Geometry check sheet. Reference: the model listing, model coordinates, mm. Face numbers are marked on the shaded views. A direction names the side the tool comes from. Give positions to 0.01 mm unless a question says otherwise; leave off trailing zeros. Order: outer loops, then holes, each group sorted by start corner. A loop starts at its lowest first (then second) coordinate and runs counter-clockwise, first axis right, second up. Notation, with made-up numbers: (65, 17) - (119, 17) arc R18 ccw to (119, 52) - close; hole circle Ø6 at (44, 24). An arc over 180 degrees is marked (long way). Put each result on its own line as item: value. Start each with the question number.
```python
from build123d import *

# Parameters (mm, degrees)
SKETCH1_W           = 40.5
SKETCH1_H           = 28.26
BOSS_EXTRUDE1_DEPTH = 2
SKETCH2_R           = 44
CUT_EXTRUDE1_DEPTH  = 1.8
CHAMFER1_SIZE       = 4.945459355
CHAMFER1_SIZE_2     = 1.8
CUT_EXTRUDE2_DEPTH  = 43.940737069


with BuildPart() as part:
    # Sketch1 → Boss-Extrude1 (new body)
    with BuildSketch(Plane(origin=(0, 0, 0), x_dir=(1, 0, 0), z_dir=(0, 1, 0))):
        Rectangle(SKETCH1_W, SKETCH1_H)
    extrude(amount=BOSS_EXTRUDE1_DEPTH)

    # Sketch2 → Cut-Extrude1 (cut)
    with BuildSketch(Plane(origin=(0, 2, 0), x_dir=(1, 0, 0), z_dir=(0, 1, 0))):
        with Locations((0, 51.13)):
            Circle(SKETCH2_R)
    extrude(amount=-CUT_EXTRUDE1_DEPTH, mode=Mode.SUBTRACT)

    # Chamfer1
    # the kernel refuses this chamfer: 4.945459355, 1.8 mm, written as the material it takes off along each edge
    with BuildSketch(Plane(origin=(0, 2, -51.13), x_dir=(-0.6960446295726113, 0, 0.7179985192485611), z_dir=(-0.7179985192485611, 0, -0.6960446295726113))) as chamfer1_piece_1_section:
        Polygon((44 + CHAMFER1_SIZE, 0), (44, -CHAMFER1_SIZE_2), (44, 0), align=None)
    chamfer1_piece_1 = revolve(axis=Axis((0, 2, -51.13), (0, 1, 0)), revolution_arc=88.221038487, mode=Mode.PRIVATE)
    chamfer1_piece_1 = split(chamfer1_piece_1, bisect_by=Plane(origin=(0, 0.2, -4.588848893), z_dir=(0, 1, 0)), keep=Keep.TOP, mode=Mode.PRIVATE)
    add(chamfer1_piece_1, mode=Mode.SUBTRACT)

    # Sketch3 → Cut-Extrude2 (cut, through all)
    with BuildSketch(Plane(origin=(20.25, 0, 0), x_dir=(0, 0, -1), z_dir=(1, 0, 0))):
        Polygon((-12.38, 2), (-11.63, 1.25), (-10.88, 2), (-10.88, 3.484474426), (-12.38, 3.484474426), align=None)
    extrude(amount=-CUT_EXTRUDE2_DEPTH, mode=Mode.SUBTRACT)


solid = part.part
```
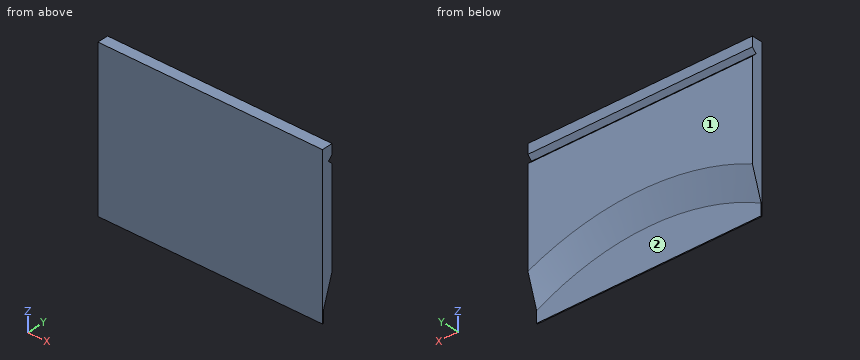
Item 1: Gauge pin test, flat end, axial feed: pin 1 Ø5.5 at (x, z) = (9, -11.5) entering from +Y. Record the tip position at first contact, or that the pin passes through.
Item 2: Set-up check for the marked faces 1 and 2: record each of +Z, -Z, +X, -X, +Y, -Y from which the full face is reachable in a straight line by a thin tool's end or side.
Item 3: Cross-section at A-A (y = 1.65). Enter the section's corners in (x, z).
Item 4: Thickness scan on line 1 along Y through (x, z) = (17.5, -12.25); line 2 along Y through (x, z) = (7.5, 11.5). Record the ranges inside material, lowest first.
Recorded:
1. pin 1: stops at y = 0.2
2. face 1: +Z, -Z, +X, -X, +Y
2. face 2: -Z, +Y
3. outline: (-20.25, -7.63) arc R47.98 cw to (20.25, -7.63) - (20.25, 11.23) - (-20.25, 11.23) - close; (-20.25, 12.03) - (20.25, 12.03) - (20.25, 14.13) - (-20.25, 14.13) - close
4. line 1: y = 0 to 0.2
4. line 2: y = 0 to 1.38
